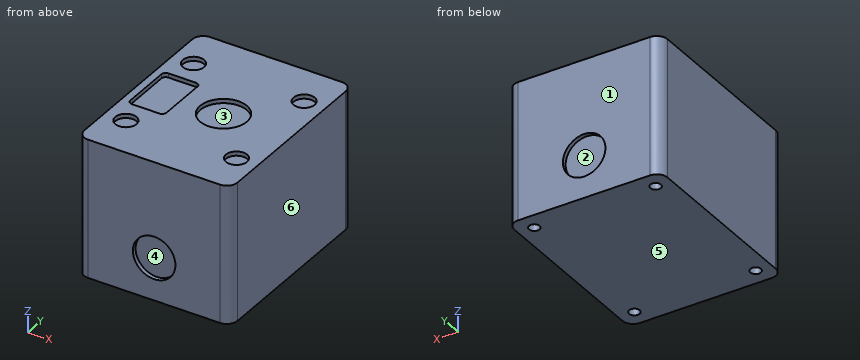
from build123d import *

# Parameters (mm, degrees)
F1_DEPTH = 65
F2_R     = 11
F2_R_2   = 5
F3_DEPTH = 2
F4_R     = 10
F5_DEPTH = 2
F6_R     = 10
F7_DEPTH = 2
F8_R     = 2.5
F9_DEPTH = 25


with BuildPart() as f1:
    # F0 (on Top) → F1 (new body)
    with BuildSketch(Plane.XY):
        with BuildLine():
            Line((-31, -45), (31, -45))
            ThreePointArc((31, -45), (34.535534, -43.535534), (36, -40))
            Line((36, -40), (36, 40))
            ThreePointArc((36, 40), (34.535534, 43.535534), (31, 45))
            Line((31, 45), (-31, 45))
            ThreePointArc((-31, 45), (-34.535534, 43.535534), (-36, 40))
            Line((-36, 40), (-36, -40))
            ThreePointArc((-36, -40), (-34.535534, -43.535534), (-31, -45))
        make_face()
    extrude(amount=F1_DEPTH)

    # F2 (on face) → F3 (cut)
    with BuildSketch(Plane.XY.offset(65)):
        with Locations((4, 0)):
            Circle(F2_R)
        with BuildLine():
            ThreePointArc((-15.5, 11.5), (-16.085786, 12.914214), (-17.5, 13.5))
            Line((-17.5, 13.5), (-30.5, 13.5))
            ThreePointArc((-30.5, 13.5), (-31.914214, 12.914214), (-32.5, 11.5))
            Line((-32.5, 11.5), (-32.5, -11.5))
            ThreePointArc((-32.5, -11.5), (-31.914214, -12.914214), (-30.5, -13.5))
            Line((-30.5, -13.5), (-17.5, -13.5))
            ThreePointArc((-17.5, -13.5), (-16.085786, -12.914214), (-15.5, -11.5))
            Line((-15.5, -11.5), (-15.5, 11.5))
        make_face()
        with Locations((-26, 25)):
            Circle(F2_R_2)
        with Locations((26, 25)):
            Circle(F2_R_2)
        with Locations((26, -25)):
            Circle(F2_R_2)
        with Locations((-26, -25)):
            Circle(F2_R_2)
    extrude(amount=-F3_DEPTH, mode=Mode.SUBTRACT)

    # F4 (on face) → F5 (cut)
    with BuildSketch(Plane(origin=(0, 45, 0), x_dir=(-1, 0, 0), z_dir=(0, 1, 0))):
        with Locations((0, 20)):
            Circle(F4_R)
    extrude(amount=-F5_DEPTH, mode=Mode.SUBTRACT)

    # F6 (on face) → F7 (cut)
    with BuildSketch(Plane.XZ.offset(45)):
        with Locations((0, 20)):
            Circle(F6_R)
    extrude(amount=-F7_DEPTH, mode=Mode.SUBTRACT)

    # F8 (on face) → F9 (cut)
    with BuildSketch(Plane(origin=(0, 0, 0), x_dir=(1, 0, 0), z_dir=(0, 0, -1))):
        with Locations((28.5, -37)):
            Circle(F8_R)
        with Locations((-28.5, -37)):
            Circle(F8_R)
        with Locations((-28.5, 37)):
            Circle(F8_R)
        with Locations((28.5, 37)):
            Circle(F8_R)
    extrude(amount=-F9_DEPTH, mode=Mode.SUBTRACT)


solid = f1.part
Part model, mm, in its own coordinate system. Face numbers are marked on the shaded views. A direction names the side the tool comes from. Round coordinates to 2 decimals unless told otherwise and drop trailing zeros. Loops run counter-clockwise (first coordinate to the right, second up) from the corner with the lowest first, then second, coordinate; pieces in that order, holes last. Notation, with made-up numbers: (-21.75, -2) - (34.25, -2) arc R35 cw to (34.25, 31) - close; hole circle Ø5 at (73.5, -9.75). An arc over 180 degrees is marked (long way). Answer as a JSON object with one key per item and string values.
Item 1: Band-saw the part on D-D on x = -27.5. List the corners of the cut face in (y, z).
Output:
{"outline": "(-45, 0) - (-39.29, 0) - (-39.29, 25) - (-34.71, 25) - (-34.71, 0) - (34.71, 0) - (34.71, 25) - (39.29, 25) - (39.29, 0) - (45, 0) - (45, 65) - (29.77, 65) - (29.77, 63) - (20.23, 63) - (20.23, 65) - (13.5, 65) - (13.5, 63) - (-13.5, 63) - (-13.5, 65) - (-20.23, 65) - (-20.23, 63) - (-29.77, 63) - (-29.77, 65) - (-45, 65) - close"}
Item 2: Pull direction Z, two halves, no side cores. Call the marked faces 4, 5 and 6: pulls with the +Z half, pulls with the -Z half, needs draft (parallel to the pull), parting line crosses it, or undercut.
Output:
{"face 4": "undercut", "face 5": "pulls with the -Z half", "face 6": "needs draft"}
Item 3: Band-saw the part on C-C on x = 29.5. List the corners of the cut face in (y, z).
Output:
{"outline": "(-45, 0) - (-39.29, 0) - (-39.29, 25) - (-34.71, 25) - (-34.71, 0) - (34.71, 0) - (34.71, 25) - (39.29, 25) - (39.29, 0) - (45, 0) - (45, 65) - (28.57, 65) - (28.57, 63) - (21.43, 63) - (21.43, 65) - (-21.43, 65) - (-21.43, 63) - (-28.57, 63) - (-28.57, 65) - (-45, 65) - close"}
Item 4: Band-saw the part on B-B on x = 5.5. List the corners of the cut face in (y, z), plus the area to 3 significant figures.
Output:
{"outline": "(-45, 0) - (45, 0) - (45, 11.65) - (43, 11.65) - (43, 28.35) - (45, 28.35) - (45, 65) - (10.9, 65) - (10.9, 63) - (-10.9, 63) - (-10.9, 65) - (-45, 65) - (-45, 28.35) - (-43, 28.35) - (-43, 11.65) - (-45, 11.65) - close", "area": "5,740 mm2"}
Item 5: Band-saw the part on A-A on z = 17. List the corners of the cut face in (x, y), plus the area to 3 significant figures.
Output:
{"outline": "(-36, -40) arc R5 ccw to (-31, -45) - (-9.54, -45) - (-9.54, -43) - (9.54, -43) - (9.54, -45) - (31, -45) arc R5 ccw to (36, -40) - (36, 40) arc R5 ccw to (31, 45) - (9.54, 45) - (9.54, 43) - (-9.54, 43) - (-9.54, 45) - (-31, 45) arc R5 ccw to (-36, 40) - close; hole circle Ø5 at (-28.5, -37); hole circle Ø5 at (-28.5, 37); hole circle Ø5 at (28.5, -37); hole circle Ø5 at (28.5, 37)", "area": "6,300 mm2"}
Item 6: Tool access for the marked faces 1, 2 and 3: list every direction of +Z, -Z, +X, -X, +Y, -Y with a clear straight run to the whole face (end or side of a thin tool).
Output:
{"face 1": "+Z, -Z, +X, -X, +Y", "face 2": "+Y", "face 3": "+Z"}
Item 7: Wall check: L1, parallel to Y at x = -26, z = 64.45; L2, parallel to X at y = -37, z = 11; L3, parallel to Y at x = 30, z = 6. Give the ranges that are in metal, low to high.
Output:
{"L1": "-45 to -30, -20 to -13.5, 13.5 to 20, 30 to 45", "L2": "-36 to -31, -26 to 26, 31 to 36", "L3": "-45 to -39, -35 to 35, 39 to 45"}
Item 8: Pin check, flat tips, straight feed: pin 1 (5 mm diameter, centred on x = 27.5, y = -26, fed in from +Z); pin 2 (18 mm diameter, centred on x = 0, z = 20, fed in from +Y). Stop position of each tip, or through.
Output:
{"pin 1": "z = 63", "pin 2": "y = 43"}
